Work out the finished part from the listing and answer in its coordinate system (mm). Face numbers are marked on the shaded views. A direction names the side the tool comes from. Coordinates: 2 decimals unless noted, no trailing zeros. Order: outer loops, then holes, each group sorted by start corner. A loop starts at its lowest first (then second) coordinate and runs counter-clockwise, first axis right, second up. Notation, with made-up numbers: M 58,64.5 L 98,64.5 A21 cw 98,93.5 Z; hole C 47,60.25 d9. An arc over 180 degrees is marked long. Use a Markdown table: item, result.
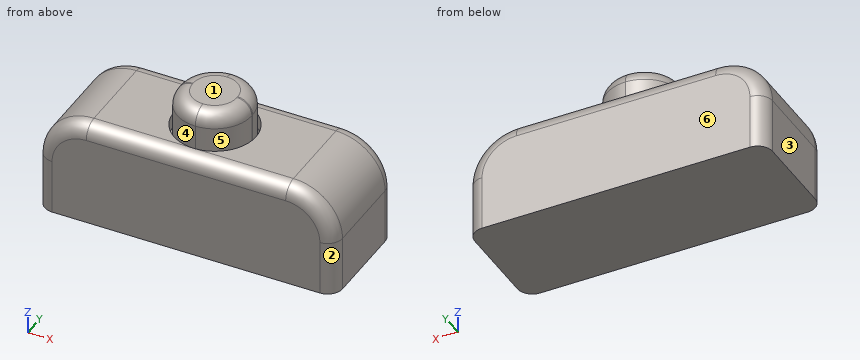
from build123d import *

# Parameters (mm, degrees)
F0_W     = 50.8
F0_H     = 19.05
F0_W_2   = 45.72
F0_H_2   = 13.97
F1_DEPTH = 12.7
F2_W     = 50.8
F2_H     = 19.05
F3_DEPTH = 2.54
F5_START = 0.508
F4_W     = 4.572
F4_H     = 2.794
F4_W_2   = 12.7
F4_H_2   = 5.08
F4_H_3   = 3.81
F5_DEPTH = 12.954
F6_R     = 6.34999
F7_W     = 50.8
F7_H     = 19.05
F7_R     = 6.985
F8_DEPTH = 2.54
F9_R     = 2.54
F10_R    = 8.382
F11_R    = 2.54


# Not quite as in the source:
# - a fillet or chamfer is up to 0.001 mm smaller than in the source, because OpenCascade refuses the exact size


with BuildPart() as f1:
    # F0 (on Top) → F1 (new body)
    with BuildSketch(Plane.XY):
        Rectangle(F0_W, F0_H)
        Rectangle(F0_W_2, F0_H_2, mode=Mode.SUBTRACT)
    extrude(amount=F1_DEPTH)

    # F2 (on face) → F3 (join)
    with BuildSketch(Plane(origin=(0, 0, 0), x_dir=(1, 0, 0), z_dir=(0, 0, -1))):
        Rectangle(F2_W, F2_H)
    extrude(amount=F3_DEPTH)

    # F4 (on face) → F5 (join)
    with BuildSketch(Plane.XZ.offset(-6.985).offset(F5_START)):
        Polygon((-25.4, 0.254), (-25.4, -2.54), (20.828, -2.54), (20.828, 0.254), (-20.828, 0.254), align=None)
        with Locations((23.114, -1.143)):
            Rectangle(F4_W, F4_H)
        with BuildLine():
            Line((-20.828, 0.254), (20.828, 0.254))
            Line((20.828, 0.254), (20.828, 0.508))
            ThreePointArc((20.828, 0.508), (19.7166563034, 0.9891715443), (19.3070802744, 2.1288462099))
            Line((19.3070802744, 2.1288462099), (5.08, 7.62))
            Line((5.08, 7.62), (-5.08, 7.62))
            Line((-5.08, 7.62), (-19.3070802744, 2.1288462099))
            ThreePointArc((-19.3070802744, 2.1288462099), (-19.3047702633, 2.0804475914), (-19.304, 2.032))
            ThreePointArc((-19.304, 2.032), (-19.7503692655, 0.9543692655), (-20.828, 0.508))
            Line((-20.828, 0.508), (-20.828, 0.254))
        make_face()
        with BuildLine():
            ThreePointArc((19.3070802744, 2.1288462099), (19.7166563034, 0.9891715443), (20.828, 0.508))
            Line((20.828, 0.508), (20.828, 2.032))
            Line((20.828, 2.032), (19.558, 2.032))
            Line((19.558, 2.032), (19.3070802744, 2.1288462099))
        make_face()
        with BuildLine():
            Line((20.828, 2.032), (20.828, 0.508))
            ThreePointArc((20.828, 0.508), (21.9056307345, 0.9543692655), (22.352, 2.032))
            ThreePointArc((22.352, 2.032), (21.7251962822, 3.2639151071), (20.3603794867, 3.4824851104))
            Line((20.3603794867, 3.4824851104), (20.828, 3.302))
            Line((20.828, 3.302), (20.828, 2.032))
        make_face()
        with BuildLine():
            ThreePointArc((-20.3603794867, 3.4824851104), (-22.3335091013, 2.2686819509), (-20.828, 0.508))
            Line((-20.828, 0.508), (-20.828, 2.032))
            Line((-20.828, 2.032), (-20.828, 3.302))
            Line((-20.828, 3.302), (-20.3603794867, 3.4824851104))
        make_face()
        with BuildLine():
            Line((-20.828, 2.032), (-20.828, 0.508))
            ThreePointArc((-20.828, 0.508), (-19.7503692655, 0.9543692655), (-19.304, 2.032))
            ThreePointArc((-19.304, 2.032), (-19.3047702633, 2.0804475914), (-19.3070802744, 2.1288462099))
            Line((-19.3070802744, 2.1288462099), (-19.558, 2.032))
            Line((-19.558, 2.032), (-20.828, 2.032))
        make_face()
        with BuildLine():
            Line((19.558, 2.032), (20.828, 2.032))
            Line((20.828, 2.032), (20.828, 3.302))
            Line((20.828, 3.302), (20.3603794867, 3.4824851104))
            ThreePointArc((20.3603794867, 3.4824851104), (19.6252291828, 2.9679051027), (19.3070802744, 2.1288462099))
            Line((19.3070802744, 2.1288462099), (19.558, 2.032))
        make_face()
        with BuildLine():
            Line((5.08, 7.62), (19.3070802744, 2.1288462099))
            ThreePointArc((19.3070802744, 2.1288462099), (19.6252291828, 2.9679051027), (20.3603794867, 3.4824851104))
            Line((20.3603794867, 3.4824851104), (6.35, 8.89))
            Line((6.35, 8.89), (6.35, 7.62))
            Line((6.35, 7.62), (5.08, 7.62))
        make_face()
        with BuildLine():
            Line((-20.828, 3.302), (-20.828, 2.032))
            Line((-20.828, 2.032), (-19.558, 2.032))
            Line((-19.558, 2.032), (-19.3070802744, 2.1288462099))
            ThreePointArc((-19.3070802744, 2.1288462099), (-19.6252291828, 2.9679051027), (-20.3603794867, 3.4824851104))
            Line((-20.3603794867, 3.4824851104), (-20.828, 3.302))
        make_face()
        with BuildLine():
            Line((-6.35, 8.89), (-20.3603794867, 3.4824851104))
            ThreePointArc((-20.3603794867, 3.4824851104), (-19.6252291828, 2.9679051027), (-19.3070802744, 2.1288462099))
            Line((-19.3070802744, 2.1288462099), (-5.08, 7.62))
            Line((-5.08, 7.62), (-6.35, 7.62))
            Line((-6.35, 7.62), (-6.35, 8.89))
        make_face()
        Polygon((-5.08, 7.62), (5.08, 7.62), (6.35, 7.62), (6.35, 8.89), (6.35, 12.7), (-6.35, 12.7), (-6.35, 8.89), (-6.35, 7.62), align=None)
        with Locations((0, 15.24)):
            Rectangle(F4_W_2, F4_H_2)
        with Locations((0, 19.685)):
            Rectangle(F4_W_2, F4_H_3)
    extrude(amount=F5_DEPTH)

    # F6 (radius 6.35 in the source; OpenCascade refuses exactly that, so slightly less here)
    f6_edges = [f1.edges().sort_by_distance(p)[0] for p in [
        (-6.35, -6.477, 15.24),
        (6.35, -6.477, 15.24),
        (6.35, 6.477, 15.24),
        (-6.35, 6.477, 15.24),
    ]]
    fillet(f6_edges, radius=F6_R)

    # F7 (on face) → F8 (join)
    with BuildSketch(Plane.XY.offset(12.7)):
        Rectangle(F7_W, F7_H)
        Circle(F7_R, mode=Mode.SUBTRACT)
    extrude(amount=F8_DEPTH)

    # F9
    f9_edges = [f1.edges().sort_by_distance(p)[0] for p in [
        (4.490131, -4.617131, 21.59),
    ]]
    fillet(f9_edges, radius=F9_R)

    # F10
    f10_edges = [f1.edges().sort_by_distance(p)[0] for p in [
        (25.4, 0, 15.24),
        (-25.4, 0, 15.24),
    ]]
    fillet(f10_edges, radius=F10_R)

    # F11
    f11_edges = [f1.edges().sort_by_distance(p)[0] for p in [
        (0, 9.525, 15.24),
        (0, -9.525, 15.24),
        (-22.944969, -9.525, 12.784969),
        (-22.944969, 9.525, 12.784969),
        (-25.4, 9.525, 2.159),
        (-25.4, -9.525, 2.159),
        (25.4, 9.525, 2.159),
        (22.944969, 9.525, 12.784969),
        (22.944969, -9.525, 12.784969),
        (25.4, -9.525, 2.159),
    ]]
    fillet(f11_edges, radius=F11_R)


solid = f1.part
1. For the marked faces 5 and 6, determine the directions among +Z, -Z, +X, -X, +Y, -Y from which every point of the face is accessible in a straight line to the end or side of a thin tool.
Answers below:
| item | result |
|---|---|
| face 5 | +Z |
| face 6 | +Z, -Z, +X, -X, +Y |
2. Section C-C on z = 2.75 is taken. Determine the outline of the cut face in (x, y) (3 decimals), then the cut area to 3 significant figures.
Answers below:
| item | result |
|---|---|
| outline | M -25.4,-6.985 A2.54 ccw -22.86,-9.525 L 22.86,-9.525 A2.54 ccw 25.4,-6.985 L 25.4,6.985 A2.54 ccw 22.86,9.525 L -22.86,9.525 A2.54 ccw -25.4,6.985 Z; M -22.172,-6.477 L 22.172,-6.477 L 22.172,6.477 L -22.172,6.477 Z; hole M -22.86,-6.985 L 22.86,-6.985 L 22.86,6.985 L -22.86,6.985 Z |
| area | 898 mm² |
3. Find the intervals of material crossed by probe 1 along Y at (x, z) = (16, 4) (3 decimals); probe 2 along Y at (x, z) = (0, 13.45) (3 decimals); probe 3 along X at (y, z) = (0, 14.25) (3 decimals), in increasing order.
Answers below:
| item | result |
|---|---|
| probe 1 | -9.525 to -6.985, -6.477 to 6.477, 6.985 to 9.525 |
| probe 2 | -9.412 to -6.985, -6.477 to 6.477, 6.985 to 9.412 |
| probe 3 | -20.97 to -6.985, -6.35 to 6.35, 6.985 to 20.97 |
4. Section D-D on y = 8.5 is taken. Determine the outline of the cut face in (x, z), then the cut area to 3 significant figures.
Answers below:
| item | result |
|---|---|
| outline | M -24.9,-2.54 L 24.9,-2.54 L 24.9,6.86 A7.88 ccw 17.02,14.74 L -17.02,14.74 A7.88 ccw -24.9,6.86 Z |
| area | 834 mm² |
5. Section B-B on x = 8 is taken. Determine the outline of the cut face in (y, z) (3 decimals).
Answers below:
| item | result |
|---|---|
| outline | M -9.525,-2.54 L 9.525,-2.54 L 9.525,12.7 A2.54 ccw 6.985,15.24 L -6.985,15.24 A2.54 ccw -9.525,12.7 Z; hole M -6.985,0 L -6.477,0 L -6.477,8.253 L 6.477,8.253 L 6.477,0 L 6.985,0 L 6.985,12.7 L -6.985,12.7 Z |
6. Flat-ended cylindrical pins translate along their axes: P1, Ø1, axis at x = 22, y = -2, coming from the +Z side; P2, Ø8, axis at x = -13.5, y = 6, coming from the +Z side; P3, Ø3, axis at y = -2.5, z = 12.5, coming from the +X side. Find the tip coordinate at first contact, or state that the pin passes through.
Answers below:
| item | result |
|---|---|
| P1 | z = 13.94 |
| P2 | z = 15.24 |
| P3 | x = 24.31 |
7. For a pull along X with two mould halves and no side action, classify the marked faces 1, 2, 3 and 4 as +X half, -X half, draft (parallel to the pull), parting line (faces both ways), or undercut.
Answers below:
| item | result |
|---|---|
| face 1 | draft |
| face 2 | +X half |
| face 3 | -X half |
| face 4 | undercut |
